```python
from build123d import *

# Parameters (mm, degrees)
F0_W     = 193.675
F0_H     = 69.85
F1_DEPTH = 9.525
F2_W     = 6.35
F2_H     = 6.35
F3_DEPTH = 2.54
F4_W     = 6.35
F4_H     = 6.35
F5_DEPTH = 77.47


with BuildPart() as f1:
    # F0 (on Top) → F1 (new body)
    with BuildSketch(Plane.XY):
        Polygon((222.25, -101.6), (222.25, 101.6), (-222.25, 101.6), (-222.25, -12.7), (-222.25, -101.6), align=None)
        with Locations((-106.3625, -47.625)):
            Rectangle(F0_W, F0_H, mode=Mode.SUBTRACT)
        with Locations((106.3625, -47.625)):
            Rectangle(F0_W, F0_H, mode=Mode.SUBTRACT)
        with Locations((-106.3625, 47.625)):
            Rectangle(F0_W, F0_H, mode=Mode.SUBTRACT)
        with Locations((106.3625, 47.625)):
            Rectangle(F0_W, F0_H, mode=Mode.SUBTRACT)
    extrude(amount=F1_DEPTH)

    # F2 (on face) → F3 (join)
    with BuildSketch(Plane.XY.offset(9.525)):
        with Locations((-212.725, 0)):
            Rectangle(F2_W, F2_H)
        with Locations((212.725, 0)):
            Rectangle(F2_W, F2_H)
        Rectangle(F2_W, F2_H)
    extrude(amount=F3_DEPTH)

    # F4 (on face) → F5 (join)
    with BuildSketch(Plane.XY.offset(12.065)):
        Rectangle(F4_W, F4_H)
        with Locations((212.725, 0)):
            Rectangle(F4_W, F4_H)
        with Locations((-212.725, 0)):
            Rectangle(F4_W, F4_H)
    extrude(amount=F5_DEPTH)


solid = f1.part
```
Verification items for the finished model (mm, model axes). A direction names the side the tool comes from. Give positions to 0.01 mm unless a question says otherwise; leave off trailing zeros. Order: outer loops, then holes, each group sorted by start corner. A loop starts at its lowest first (then second) coordinate and runs counter-clockwise, first axis right, second up. Notation, with made-up numbers: M 18.25,83 L 52.25,83 A22 cw 52.25,114 Z; hole C 19,-30 d3. An arc over 180 degrees is marked long. Answer in a Markdown table with one row per item. Add a question column.
Item 1: Section check B-B, the plane z = 48.5. Enter the section's corners in (x, y) (3 decimals), and give its area (3 significant figures).
Item 2: Mould release check, pull along Y, two halves, no side actions. Record for faces 1 (the flat face through (9.525, 47, 5)), 2 (the flat face through (-222.25, 1, 5)), 3 (the flat face through (3, 101.6, 5)): released by +Y, released by -Y, zero draft, split by the parting line, or undercut.
Item 3: Section check C-C, the plane y = 88. Enter the section's corners in (x, z) (3 decimals).
Item 4: Scan lines: probe 1 along Z at (x, y) = (130.5, -85.5) (3 decimals); probe 2 along Y at (x, z) = (-2, 57.5) (3 decimals). Record each from-to range of solid material in increasing order. Write a range as from..to.
Item 5: Section check A-A, the plane y = -43.5. Enter the section's corners in (x, z) (3 decimals).
Item 6: Gauge pin test, flat ends, axial feed: pin 1 (1.9 mm diameter, centred on x = 0.5, z = 49, fed in from -Y) (3 decimals); pin 2 (2 mm diameter, centred on y = 81, z = 12, fed in from +X) (1 decimal); pin 3 (7 mm diameter, centred on y = -0.5, z = 46, fed in from -X); pin 4 (3 mm diameter, centred on y = -1, z = 36, fed in from +X). Record the tip position at first contact, or that the pin passes through.
Item 7: Tool access check on faces 4 (the flat face through (105, 12.7, 5)), 5 (the flat face through (-3, 1, 0)). Record the directions out of +Z, -Z, +X, -X, +Y, -Y that give a thin tool (end or side, any length) a straight path to the whole face; none if there is none.
Filled sheet:
| question | item | result |
|---|---|---|
| 1 | outline | M -215.9,-3.175 L -209.55,-3.175 L -209.55,3.175 L -215.9,3.175 Z; M -3.175,-3.175 L 3.175,-3.175 L 3.175,3.175 L -3.175,3.175 Z; M 209.55,-3.175 L 215.9,-3.175 L 215.9,3.175 L 209.55,3.175 Z |
| 1 | area | 121 mm^2 |
| 2 | face 1 | undercut |
| 2 | face 2 | zero draft |
| 2 | face 3 | released by +Y |
| 3 | outline | M -222.25,0 L 222.25,0 L 222.25,9.525 L -222.25,9.525 Z |
| 4 | probe 1 | z = 0..9.525 |
| 4 | probe 2 | y = -3.175..3.175 |
| 5 | outline | M -222.25,0 L -203.2,0 L -203.2,9.525 L -222.25,9.525 Z; M -9.525,0 L 9.525,0 L 9.525,9.525 L -9.525,9.525 Z; M 203.2,0 L 222.25,0 L 222.25,9.525 L 203.2,9.525 Z |
| 6 | pin 1 | stops at y = -3.175 |
| 6 | pin 2 | passes through |
| 6 | pin 3 | stops at x = -215.9 |
| 6 | pin 4 | stops at x = 215.9 |
| 7 | face 4 | +Z, -Z |
| 7 | face 5 | -Z, +X, -X, +Y, -Y |
